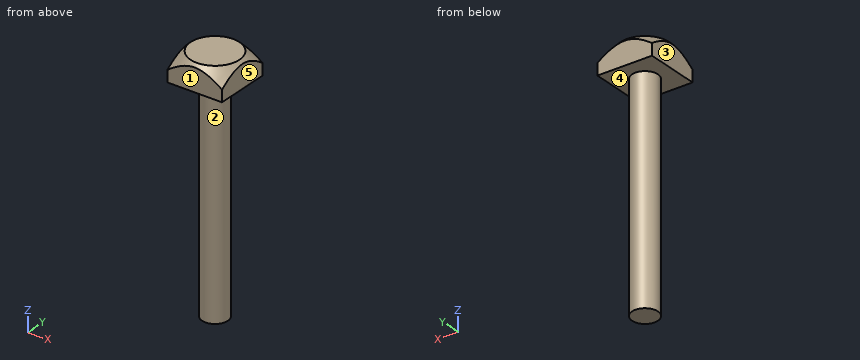
from build123d import *

# Parameters (mm, degrees)
SKETCH1_W           = 19
SKETCH1_H           = 19
BOSS_EXTRUDE1_DEPTH = 9
SKETCH2_OUTSIDE_W   = 44.668
SKETCH2_OUTSIDE_H   = 44.668
SKETCH2_OUTSIDE_R   = 8.492914758
CUT_EXTRUDE1_DEPTH  = 9
CUT_EXTRUDE1_DRAFT  = -45
SKETCH3_R           = 4.5
BOSS_EXTRUDE2_DEPTH = 76


with BuildPart() as part:
    # Sketch1 → Boss-Extrude1 (new body)
    with BuildSketch(Plane.XY):
        Rectangle(SKETCH1_W, SKETCH1_H)
    extrude(amount=BOSS_EXTRUDE1_DEPTH)


with BuildPart() as cut_extrude1_tool:
    # Sketch2 outside → Cut-Extrude1 (with draft: the straight prism first)
    with BuildSketch(Plane.XY.offset(9)):
        Rectangle(SKETCH2_OUTSIDE_W, SKETCH2_OUTSIDE_H)
        Circle(SKETCH2_OUTSIDE_R, mode=Mode.SUBTRACT)
    extrude(amount=-CUT_EXTRUDE1_DEPTH)
    # Cut-Extrude1: the draft: its side faces are tilted about the plane it starts from
    cut_extrude1_sides = [cut_extrude1_tool.faces().sort_by_distance(p)[0] for p in [
        (0, -22.334, 4.5),
        (22.334, 0, 4.5),
        (0, 22.334, 4.5),
        (-22.334, 0, 4.5),
        (-8.492914758, 0, 4.5),
    ]]
    draft(cut_extrude1_sides, Plane.XY.offset(9), CUT_EXTRUDE1_DRAFT)


with BuildPart() as part_1:
    add(part.part)

    # Cut-Extrude1: cut by cut_extrude1_tool
    add(cut_extrude1_tool.part, mode=Mode.SUBTRACT)

    # Sketch3 → Boss-Extrude2 (add)
    with BuildSketch(Plane(origin=(0, 0, 0), x_dir=(-1, 0, 0), z_dir=(0, 0, -1))):
        with Locations(Location((0, 0, 0), (0, 0, 180))):  # turned: the seam where the file's is
            Circle(SKETCH3_R)
    extrude(amount=BOSS_EXTRUDE2_DEPTH)


solid = part_1.part
CAD build for the part. Positions are in the model's coordinates, mm. Face numbers are marked on the shaded views. A direction names the side the tool comes from. Coordinates: 2 decimals unless noted, no trailing zeros. Write each loop counter-clockwise with the first axis right and the second up, starting at its lowest first coordinate (ties: lowest second). Pieces come first, ordered by that corner, then holes. Notation, with made-up numbers: M 44,8 L 72,8 A20 cw 72,25 Z; hole C 36.25,55.25 d9. An arc over 180 degrees is marked long. Answer as a JSON object with one key per item and string values. Group by question number.
1) Pin check, flat tips, straight feed: pin 1 Ø5 at (y, z) = (6, -64.5) entering from +X; pin 2 Ø3 at (x, z) = (4, -55) entering from +Y; pin 3 Ø5 at (x, z) = (-3, -10) entering from +Y. Stop position of each tip, or through.
2) Mould opens along X. For the marked faces 1, 2 and 3 say: +X half, -X half, draft (parallel to the pull), parting line (faces both ways), or undercut.
3) Saw through at C-C (z = -64.5). Write the cut outline in (x, y).
4) Saw through at A-A (x = 0). Write the cut outline in (y, z).
5) Wall check: line 1 (Z direction, x = 5.75, y = 0); line 2 (Z direction, x = 5, y = 7.5); line 3 (X direction, y = -1.5, z = -71.5). Give the ranges that are in metal, low to high. Write a range as from..to.
6) Tool access for the marked faces 4 and 5: list every direction of +Z, -Z, +X, -X, +Y, -Y with a clear straight run to the whole face (end or side of a thin tool).
Values follow:
{
 "1": {"pin 1": "stops at x = 2.83", "pin 2": "stops at y = 3.74", "pin 3": "stops at y = 4.47"},
 "2": {"face 1": "draft", "face 2": "parting line", "face 3": "-X half"},
 "3": {"outline": "C 0,0 d9"},
 "4": {"outline": "M -9.5,0 L -4.5,0 L -4.5,-76 L 4.5,-76 L 4.5,0 L 9.5,0 L 9.5,7.99 L 8.49,9 L -8.49,9 L -9.5,7.99 Z"},
 "5": {"line 1": "z = 0..9", "line 2": "z = 0..8.48", "line 3": "x = -4.24..4.24"},
 "6": {"face 4": "-Z", "face 5": "+Z, -Z, +X, +Y, -Y"}
}
